Autodesk Inventor part; units mm, degrees
ref_plane "YZ Plane" through (0, 0, 0) normal (1, 0, 0) x (0, 1, 0)
ref_plane "XZ Plane" through (0, 0, 0) normal (0, 1, 0) x (-1, 0, 0)
ref_plane "XY Plane" through (0, 0, 0) normal (0, 0, 1) x (1, 0, 0)
sketch "Sketch1" plane through (0, 0, 0) normal (1, 0, 0) x (0, 1, 0)
  line L0 (0, 0) -> (25.4, 0)
  line L1 (25.4, 0) -> (25.4, -50.8)
  line L2 (25.4, -50.8) -> (0, -50.8)
  line L3 (0, -50.8) -> (0, 0)
  line L4 (3.175, -3.175) -> (22.225, -3.175)
  line L5 (22.225, -3.175) -> (22.225, -47.625)
  line L6 (22.225, -47.625) -> (3.175, -47.625)
  line L7 (3.175, -47.625) -> (3.175, -3.175)
  dimension "d0" = 25.4
  dimension "d1" = 50.8
  dimension "d2" = 19.05
  dimension "d3" = 44.45
  dimension "d4" = 3.175
  dimension "d5" = 3.175
extrude "Extrusion1" add sketch "Sketch1" along normal blind 469.9
sketch "Sketch2" plane through (0, 25.4, 0) normal (0, 1, 0) x (1, 0, 0)
  line L0 (0, 0) -> (0, 50.8)
  line L1 (0, 0) -> (469.9, 0)
  line L2 (469.9, 50.8) -> (469.9, 0)
  line L3 (0, 50.8) -> (469.9, 50.8)
  point P0 (12.7, 12.7)
  point P1 (12.7, 38.1)
  point P2 (457.2, 12.7)
  point P3 (457.2, 38.1)
  dimension "d8" = 12.7
  dimension "d9" = 12.7
  dimension "d10" = 12.7
  dimension "d11" = 12.7
  dimension "d12" = 12.7
  dimension "d13" = 12.7
  dimension "d14" = 12.7
  dimension "d15" = 12.7
hole "Hole1" at (12.7, 25.4, -12.7) at (12.7, 25.4, -38.1) at (457.2, 25.4, -12.7) at (457.2, 25.4, -38.1) direction (0, -1, 0) diameter 6.35 end through all
sketch "Sketch3" plane through (0, 0, 0) normal (0, 0, 1) x (1, 0, 0)
  line L0 (0, 0) -> (0, 25.4)
  line L1 (0, 0) -> (469.9, 0)
  line L2 (469.9, 25.4) -> (469.9, 0)
  line L3 (0, 25.4) -> (469.9, 25.4)
  point P0 (57.15, 12.7)
  point P1 (107.95, 12.7)
  dimension "d23" = 57.15
  dimension "d24" = 12.7
  dimension "d25" = 12.7
  dimension "d26" = 107.95
hole "Hole2" at (57.15, 12.7, 0) at (107.95, 12.7, 0) direction (0, 0, -1) diameter 6.35 end through all
properties part number "2x1 support horizontal"
Geometry check sheet. Reference: the model listing, model coordinates, mm. A direction names the side the tool comes from. Coordinates: 2 decimals unless noted, no trailing zeros. Order: outer loops, then holes, each group sorted by start corner. A loop starts at its lowest first (then second) coordinate and runs counter-clockwise, first axis right, second up. Notation, with made-up numbers: (64, 71.25) - (85, 71.25) arc R12 cw to (85, 79.25) - close; hole circle Ø7 at (-6, -39). An arc over 180 degrees is marked (long way). Use one line per item in the form item = value.
1. Scan lines: line 1 (Z direction, x = 457.2, y = 23.9) (3 decimals); line 2 (X direction, y = 12.7, z = -2.2) (3 decimals); line 3 (X direction, y = 2.55, z = -38.1) (3 decimals). Record each from-to range of solid material in increasing order.
Here are the results:
line_1 = -50.8 to -41.275, -34.925 to -15.875, -9.525 to 0
line_2 = 0 to 53.975, 60.325 to 104.775, 111.125 to 469.9
line_3 = 0 to 9.525, 15.875 to 454.025, 460.375 to 469.9
2. Gauge pin test, flat end, axial feed: pin 1 (4 mm diameter, centred on x = 107.95, y = 12.7, fed in from +Z). Record the tip position at first contact, or that the pin passes through.
Here are the results:
pin_1 = through
3. Access from +Z, -Z, +X, -X, +Y, -Y to the whole of each face (thin tool, end or side, straight path). Record for faces 1 (the face through (232, 25.4, -25)), 2 (the face through (232, 22.225, -25)).
Here are the results:
face_1 = +Z, -Z, +X, -X, +Y
face_2 = +X, -X
4. Section check A-A (z = -31). Record the boundary of the cut face in (x, y) (3 decimals).
Here are the results:
outline = (0, 0) - (469.9, 0) - (469.9, 3.175) - (0, 3.175) - close; (0, 22.225) - (469.9, 22.225) - (469.9, 25.4) - (0, 25.4) - close
5. Section check B-B (x = 288.5). Record the boundary of the cut face in (y, z) (3 decimals), then the cut area to 3 significant figures.
Here are the results:
outline = (0, -50.8) - (25.4, -50.8) - (25.4, 0) - (0, 0) - close; hole (3.175, -47.625) - (22.225, -47.625) - (22.225, -3.175) - (3.175, -3.175) - close
area = 444 mm²
6. Draft check along Z on faces 3 (the face through (232, 13, -50.8)), 4 (the face through (0, 2, -27)), 5 (the face through (232, 13, 0)), 6 (the face through (232, 3.175, -26)). Enter one of: pulls with the +Z half, pulls with the -Z half, needs draft (parallel to the pull), parting line crosses it, or undercut.
Here are the results:
face_3 = pulls with the -Z half
face_4 = needs draft
face_5 = pulls with the +Z half
face_6 = undercut
